Can you work these out from the model? Positions are in its coordinate system, mm. Face numbers are marked on the shaded views. A direction names the side the tool comes from. Round coordinates to 2 decimals unless told otherwise and drop trailing zeros. Loops run counter-clockwise (first coordinate to the right, second up) from the corner with the lowest first, then second, coordinate; pieces in that order, holes last. Notation, with made-up numbers: M 56,-25 L 106,-25 A33 ccw 106,7 Z; hole C -15,15 d10. An arc over 180 degrees is marked long. Use a Markdown table: item, result. Add a question column.
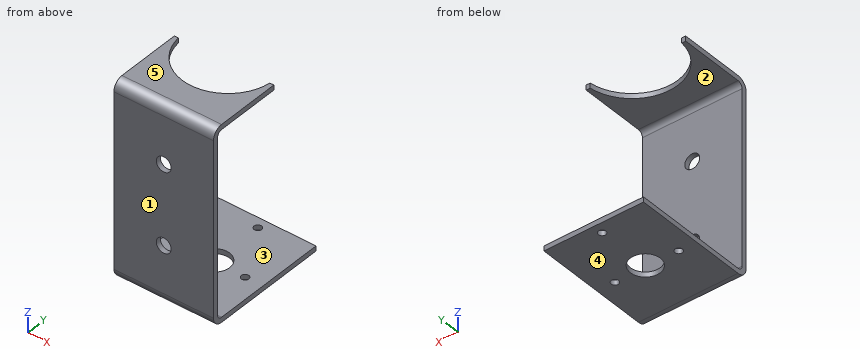
```python
from build123d import *

# Parameters (mm, degrees)
SKETCH44_W          = 40
SKETCH44_H          = 70
BOSS_EXTRUDE1_DEPTH = 2
EDGE_FLANGE6_DEPTH  = 40
SKETCH52_R          = 6
SKETCH52_R_2        = 1.5
CUT_EXTRUDE5_DEPTH  = 25
SKETCH54_R          = 3
CUT_EXTRUDE6_DEPTH  = 11
EDGE_FLANGE7_DEPTH  = 40
CUT_EXTRUDE8_START  = -10
SKETCH52_4_R        = 18.5
CUT_EXTRUDE8_DEPTH  = 84


# Sheet-metal steps are written as plain solids
with BuildPart() as part:
    # Sketch44 → Boss-Extrude1 (new body)
    with BuildSketch(Plane(origin=(0, 0, 0), x_dir=(1, 0, 0), z_dir=(0, 1, 0))):
        Rectangle(SKETCH44_W, SKETCH44_H)
    extrude(amount=BOSS_EXTRUDE1_DEPTH)

    # Edge-Flange6 section (across the edge) → Edge-Flange6 (add)
    with BuildSketch(Plane(origin=(20, 2, -37), x_dir=(0, 0, 1), z_dir=(-1, 0, 0))):
        with BuildLine():
            Line((-2, 2), (-2, 49))
            Line((-2, 49), (0, 49))
            Line((0, 49), (0, 2))
            ThreePointArc((0, 2), (0.585786438, 0.585786438), (2, 0))
            Line((2, 0), (2, -2))
            ThreePointArc((2, -2), (-0.828427125, -0.828427125), (-2, 2))
        make_face()
    extrude(amount=EDGE_FLANGE6_DEPTH)

    # Sketch52 → Cut-Extrude5 (cut)
    with BuildSketch(Plane(origin=(0, 0, -39), x_dir=(-1, 0, 0), z_dir=(0, 0, -1))):
        with Locations(Location((0, 25.347000811, 0), (0, 0, 90))):
            Circle(SKETCH52_R)
        with Locations(Location((0, 46.800736891, 0), (0, 0, 90))):
            Circle(SKETCH52_R_2)
        with Locations(Location((-12.817814142, 24.599631554, 0), (0, 0, 90))):
            Circle(SKETCH52_R_2)
        with Locations(Location((12.817814142, 24.599631554, 0), (0, 0, 90))):
            Circle(SKETCH52_R_2)
    extrude(amount=-CUT_EXTRUDE5_DEPTH, mode=Mode.SUBTRACT)

    # Sketch54 → Cut-Extrude6 (cut)
    with BuildSketch(Plane(origin=(0, 2, 0), x_dir=(1, 0, 0), z_dir=(0, 1, 0))):
        with Locations(Location((0, 16, 0), (0, 0, 270))):
            Circle(SKETCH54_R)
        with Locations(Location((0, -16, 0), (0, 0, 270))):
            Circle(SKETCH54_R)
    extrude(amount=-CUT_EXTRUDE6_DEPTH, mode=Mode.SUBTRACT)

    # Edge-Flange7 section (across the edge) → Edge-Flange7 (add)
    with BuildSketch(Plane(origin=(-20, 2, 37), x_dir=(0, 0, -1), z_dir=(1, 0, 0))):
        with BuildLine():
            Line((-2, 2), (-2, 28))
            Line((-2, 28), (0, 28))
            Line((0, 28), (0, 2))
            ThreePointArc((0, 2), (0.585786438, 0.585786438), (2, 0))
            Line((2, 0), (2, -2))
            ThreePointArc((2, -2), (-0.828427125, -0.828427125), (-2, 2))
        make_face()
    extrude(amount=EDGE_FLANGE7_DEPTH)

    # Sketch52<4> → Cut-Extrude8 (cut)
    with BuildSketch(Plane(origin=(0, 0, -39), x_dir=(-1, 0, 0), z_dir=(0, 0, -1)).offset(CUT_EXTRUDE8_START)):
        with Locations((0, 32)):
            Circle(SKETCH52_4_R)
    extrude(amount=-CUT_EXTRUDE8_DEPTH, mode=Mode.SUBTRACT)


solid = part.part
```
(1) Suppose I cut it at A-A on y = 9. List the corners of the cut face in (x, z) for me.
(2) Suppose I cut it at C-C on x = 0. List the corners of the cut face in (y, z) for me, and give its area (3 significant figures).
(3) Thinking about a two-plate mould opening in Z: for the marked faces 3, 4 and 5, which applies, released by +Z, released by -Z, zero draft, split by the parting line, or undercut?
(4) I'm going to push flat-ended pins straight in: pin 1 (12 mm diameter, centred on x = 11, z = -25.5, fed in from +Y); pin 2 (1.3 mm diameter, centred on x = -19, z = 37.5, fed in from +Y); pin 3 (3.5 mm diameter, centred on x = 0, y = 46.8, fed in from +Z). Where does each tip first touch, or does it pass through?
(5) Suppose I cut it at D-D on x = 15.5. List the corners of the cut face in (y, z) for me, and give its area (3 significant figures).
(6) If I drill on probe 1 along Z at (x, y) = (14.5, 17.5); probe 2 along Y at (x, z) = (-15.5, 12.5); probe 3 along Z at (x, y) = (-17, 33.5), over which ranges is the centre line in solid material (lowest first)? Write a range as [from, to].
(7) On a 3-axis mill with a long thin cutter (end or side, diameter ignored), from which of +Z, -Z, +X, -X, +Y, -Y can I reach the whole of each face in a straight line? I mean the marked faces 1 and 2. Say none if no direction works.
(8) Suppose I cut it at B-B on z = -16. List the corners of the cut face in (x, y) for me.
Results below:
| question | item | result |
|---|---|---|
| 1 | outline | M -20,-39 L 20,-39 L 20,-37 L -20,-37 Z; M -20,37 L 20,37 L 20,39 L -20,39 Z |
| 2 | outline | M 0,-35 A4 ccw 4,-39 L 19.35,-39 L 19.35,-37 L 4,-37 A2 cw 2,-35 L 2,-19 L 0,-19 Z; M 0,-13 L 2,-13 L 2,13 L 0,13 Z; M 0,19 L 2,19 L 2,35 A2 cw 4,37 L 13.5,37 L 13.5,39 L 4,39 A4 ccw 0,35 Z; M 31.35,-39 L 45.3,-39 L 45.3,-37 L 31.35,-37 Z; M 48.3,-39 L 51,-39 L 51,-37 L 48.3,-37 Z |
| 2 | area | 218 mm² |
| 3 | face 3 | undercut |
| 3 | face 4 | released by -Z |
| 3 | face 5 | released by +Z |
| 4 | pin 1 | stops at y = 2 |
| 4 | pin 2 | stops at y = 30 |
| 4 | pin 3 | stops at z = -37 |
| 5 | outline | M 0,-35 A4 ccw 4,-39 L 51,-39 L 51,-37 L 4,-37 A2 cw 2,-35 L 2,35 A2 cw 4,37 L 21.9,37 L 21.9,39 L 4,39 A4 ccw 0,35 Z |
| 5 | area | 289 mm² |
| 6 | probe 1 | z = [-39, -37], [37, 39] |
| 6 | probe 2 | y = [0, 2] |
| 6 | probe 3 | z = [-39, -37] |
| 7 | face 1 | +Z, -Z, +X, -X, -Y |
| 7 | face 2 | +X, -X, +Y |
| 8 | outline | M -20,0 L -3,0 L -3,2 L -20,2 Z; M 3,0 L 20,0 L 20,2 L 3,2 Z |
